Study the drawing (mm; zero at the part's minimum x, y, z) and answer. Round coordinates to 2 decimals unless told otherwise and drop trailing zeros. Write each loop counter-clockwise with the first axis right and the second up, starting at its lowest first coordinate (ties: lowest second). Pieces come first, ordered by that corner, then holes. Notation, with made-up numbers: (85.5, 84.25) -> (133.5, 84.25) arc R32 ccw to (133.5, 123.25) -> close; hole circle Ø6 at (48.5, 73.25). An arc over 180 degrees is marked (long way). Return JSON: item names as keys, results as strings.
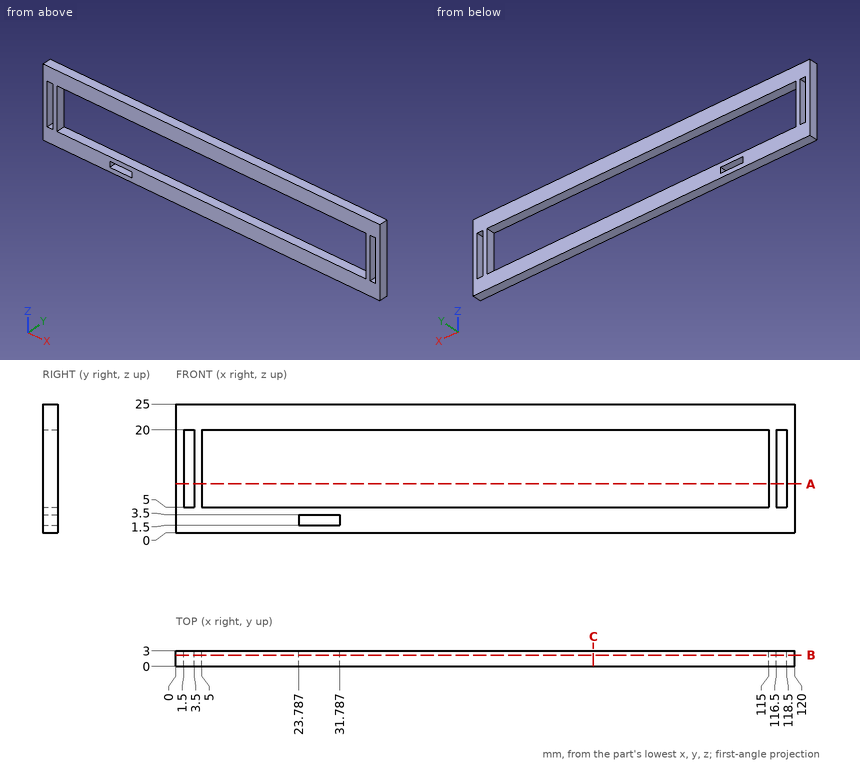
Item 1: A flat-ended cylindrical pin translates along its axis: pin 1 (1 mm diameter, centred on x = 19.5, z = 18, fed in from +Y). Find the tip coordinate at first contact, or state that the pin passes through.
Worked answers:
{"pin 1": "passes through"}
Item 2: Section B-B (y = 2.15) is taken. Give the vertices of the cut face in (x, z).
Worked answers:
{"outline": "(0, 0) -> (120, 0) -> (120, 25) -> (0, 25) -> close; hole (1.5, 5) -> (3.5, 5) -> (3.5, 20) -> (1.5, 20) -> close; hole (5, 5) -> (115, 5) -> (115, 20) -> (5, 20) -> close; hole (23.79, 1.5) -> (31.79, 1.5) -> (31.79, 3.5) -> (23.79, 3.5) -> close; hole (116.5, 5) -> (118.5, 5) -> (118.5, 20) -> (116.5, 20) -> close"}
Item 3: Section A-A (z = 9.5) is taken. Give the vertices of the cut face in (x, y).
Worked answers:
{"outline": "(0, 0) -> (1.5, 0) -> (1.5, 3) -> (0, 3) -> close; (3.5, 0) -> (5, 0) -> (5, 3) -> (3.5, 3) -> close; (115, 0) -> (116.5, 0) -> (116.5, 3) -> (115, 3) -> close; (118.5, 0) -> (120, 0) -> (120, 3) -> (118.5, 3) -> close"}
Item 4: Section C-C (x = 81) is taken. Give the vertices of the cut face in (y, z), then the cut area to 3 significant figures.
Worked answers:
{"outline": "(0, 0) -> (3, 0) -> (3, 5) -> (0, 5) -> close; (0, 20) -> (3, 20) -> (3, 25) -> (0, 25) -> close", "area": "30.0 mm2"}
Item 5: Straight lines are drawn through the part: L1, parallel to X at y = 2.05, z = 12.25; L2, parallel to Z at x = 24, y = 2.1; L3, parallel to Z at x = 49, y = 2.85. For each, find the intervals that lie inside material, in ascending order. Write a range as [from, to].
Worked answers:
{"L1": "x = [0, 1.5], [3.5, 5], [115, 116.5], [118.5, 120]", "L2": "z = [0, 1.5], [3.5, 5], [20, 25]", "L3": "z = [0, 5], [20, 25]"}
